```python
from build123d import *

# Parameters (mm, degrees)
BASE_EXTRUDE_DEPTH  = 4
SKETCH3_R           = 3
BOSS_EXTRUDE1_DEPTH = 40
CHAMFER1_SIZE       = 0.6134
FILLET1_R           = 0.25


with BuildPart() as part:
    # Sketch1 → Base-Extrude (new body)
    with BuildSketch(Plane.XY):
        Polygon((-2.886751346, 5), (2.886751346, 5), (5.773502692, 0), (2.886751346, -5), (-2.886751346, -5), (-5.773502692, 0), align=None)
    extrude(amount=BASE_EXTRUDE_DEPTH)

    # Sketch5 → Cut-Revolve1 (revolve, cut)
    with BuildSketch(Plane(origin=(0, 0, 0), x_dir=(1, 0, 0), z_dir=(0, 1, 0))):
        Polygon((-5.773502692, -4), (-5, -4), (-5.773502692, -3.553418013), align=None)
    revolve(axis=Axis((0, 0, 0), (0, 0, 1)), mode=Mode.SUBTRACT)

    # Sketch3 → Boss-Extrude1 (add)
    with BuildSketch(Plane(origin=(0, 0, 0), x_dir=(-1, 0, 0), z_dir=(0, 0, -1))):
        with Locations(Location((0, 0, 0), (0, 0, 180))):
            Circle(SKETCH3_R)
    extrude(amount=BOSS_EXTRUDE1_DEPTH)

    # Chamfer1
    chamfer1_edges = [part.edges().sort_by_distance(p)[0] for p in [
        (-3, 0, -40),
    ]]
    chamfer(chamfer1_edges, length=CHAMFER1_SIZE)

    # Fillet1
    fillet1_edges = [part.edges().sort_by_distance(p)[0] for p in [
        (-3, 0, 0),
    ]]
    fillet(fillet1_edges, radius=FILLET1_R)


solid = part.part
```
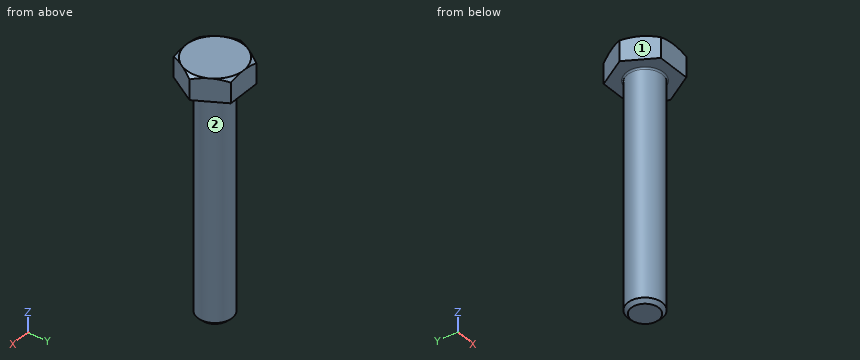
Model file for the job. Use its own axes, mm. Face numbers are marked on the shaded views. A direction names the side the tool comes from. Coordinates: 2 decimals unless noted, no trailing zeros. Loops run counter-clockwise (first coordinate to the right, second up) from the corner with the lowest first, then second, coordinate; pieces in that order, holes last. Notation, with made-up numbers: (76.25, 40.25) - (87.25, 40.25) arc R16 cw to (87.25, 61.25) - close; hole circle Ø5 at (-19.75, -18). An arc over 180 degrees is marked (long way). Answer as a JSON object with one key per item and string values. Group by question number.
(1) Flat gauge pins, fed straight in: pin 1 (2 mm diameter, centred on y = 1, z = -12.5, fed in from +X); pin 2 (1.5 mm diameter, centred on y = 3.5, z = -16, fed in from +X); pin 3 (1.5 mm diameter, centred on x = -4.5, y = 0, fed in from -Z). Where does each tip first touch, or does it go through?
(2) Cut at A-A (z = -34). Give the cut face in (x, y), then the cut area to 3 significant figures.
(3) Probe line 1 along Z through (x, y) = (4, 0); line 2 along Y through (x, z) = (0.5, -26.5); line 3 along Y through (x, z) = (-1.25, -16). List the from-to ranges inside material, lowest first.
(4) Tool access for the marked faces 1 and 2: list every direction of +Z, -Z, +X, -X, +Y, -Y with a clear straight run to the whole face (end or side of a thin tool).
Geometry says:
{
 "1": {"pin 1": "stops at x = 3", "pin 2": "stops at x = 1.2", "pin 3": "stops at z = 0"},
 "2": {"outline": "circle Ø6 at (0, 0)", "area": "28.3 mm^2"},
 "3": {"line 1": "z = 0 to 4", "line 2": "y = -2.96 to 2.96", "line 3": "y = -2.73 to 2.73"},
 "4": {"face 1": "+Z, -Z, -X, -Y", "face 2": "-Z"}
}
